The listing builds one solid part. Answer for the finished solid, in the listing's coordinates (mm). A direction names the side the tool comes from. Coordinates: 2 decimals unless noted, no trailing zeros. Order: outer loops, then holes, each group sorted by start corner. A loop starts at its lowest first (then second) coordinate and runs counter-clockwise, first axis right, second up. Notation, with made-up numbers: (-23.5, -27) -> (35.5, -27) arc R21 cw to (35.5, -22) -> close; hole circle Ø9 at (62, -14). An arc over 180 degrees is marked (long way). Return JSON: item names as keys, results as strings.
from build123d import *

# Parameters (mm, degrees)
F0_R     = 24.765
F0_R_2   = 21.082
F1_DEPTH = 30.48
F0_R_3   = 17.272
F0_R_4   = 5.55625
F2_DEPTH = 5.08
F3_SIZE2 = 4.7397045256
F3_SIZE  = 1.27
F4_SIZE  = 1.27


with BuildPart() as f1:
    # F0 (on Top) → F1 (new body)
    with BuildSketch(Plane.XY):
        Circle(F0_R)
        Circle(F0_R_2, mode=Mode.SUBTRACT)
    extrude(amount=F1_DEPTH)



with BuildPart() as f1b:
    # F0 (on Top) → F1, piece 2 (new body)
    with BuildSketch(Plane.XY):
        Circle(F0_R_3)
        Circle(F0_R_4, mode=Mode.SUBTRACT)
    extrude(amount=F1_DEPTH)


with BuildPart() as f1_1:
    add(f1.part)

    add(f1b.part)  # F2 merges F1b
    # F0 (on Top) → F2 (join)
    with BuildSketch(Plane.XY):
        Circle(F0_R_2)
        Circle(F0_R_3, mode=Mode.SUBTRACT)
    extrude(amount=F2_DEPTH)

    # F3
    f3_edges = [f1_1.edges().sort_by_distance(p)[0] for p in [
        (-24.765, 0, 30.48),
    ]]
    f3_side = f1_1.faces().sort_by_distance((-24.06454, 0, 30.48))[0]
    chamfer(f3_edges, length=F3_SIZE, length2=F3_SIZE2, reference=f3_side)

    # F4
    f4_edges = [f1_1.edges().sort_by_distance(p)[0] for p in [
        (-24.765, 0, 0),
    ]]
    chamfer(f4_edges, length=F4_SIZE)


solid = f1_1.part
1. Each of these flat-tipped pins is pushed along its axis until it touches: pin 1 Ø14.5 at (x, y) = (0, 0) entering from +Z; pin 2 Ø1.5 at (y, z) = (-15, 24.5) entering from -X; pin 3 Ø2 at (x, z) = (-17.5, 26) entering from +Y; pin 4 Ø6 at (x, z) = (-14, 5) entering from -Y. Where does it stop, or does it pass through?
Answer block:
{"pin 1": "stops at z = 30.48", "pin 2": "stops at x = -20.25", "pin 3": "stops at y = 18.44", "pin 4": "stops at y = -22.19"}
2. Determine the mould class of faces 3 (the face through (-6, 0, 0)), 4 (the face through (20.11, 6.33, 17.6)), 5 (the face through (-5.11, -23.014, 30.184)) for opening direction X: pulls with the +X half, pulls with the -X half, needs draft (parallel to the pull), parting line crosses it, or undercut.
Answer block:
{"face 3": "needs draft", "face 4": "undercut", "face 5": "parting line crosses it"}
3. The part is cut by section A-A on x = 0. Give the vertices of the cut face in (y, z) (3 decimals).
Answer block:
{"outline": "(-24.765, 1.27) -> (-23.495, 0) -> (-5.556, 0) -> (-5.556, 30.48) -> (-17.272, 30.48) -> (-17.272, 5.08) -> (-21.082, 5.08) -> (-21.082, 30.48) -> (-23.495, 30.48) -> (-24.765, 25.74) -> close; (5.556, 0) -> (23.495, 0) -> (24.765, 1.27) -> (24.765, 25.74) -> (23.495, 30.48) -> (21.082, 30.48) -> (21.082, 5.08) -> (17.272, 5.08) -> (17.272, 30.48) -> (5.556, 30.48) -> close"}
4. Consider line 1 (Y direction, x = 0, z = 17.5) (3 decimals); line 2 (X direction, y = 10.5, z = 28); line 3 (X direction, y = 10, z = 25.5). Determine where each line is inside the solid, lowest interval first. Write a range as from..to.
Answer block:
{"line 1": "y = -24.765..-21.082, -17.272..-5.556, 5.556..17.272, 21.082..24.765", "line 2": "x = -21.76..-18.28, -13.71..13.71, 18.28..21.76", "line 3": "x = -22.66..-18.56, -14.08..14.08, 18.56..22.66"}
5. The part is cut by section C-C on z = 7.5. Give the vertices of the cut face in (x, y) (1 decimal).
Answer block:
{"outline": "circle Ø49.5 at (0, 0); circle Ø34.5 at (0, 0); hole circle Ø42.2 at (0, 0); hole circle Ø11.1 at (0, 0)"}
6. For faces 1 (the face through (-8, -16, 5.08)), 2 (the face through (5.3, 1.67, 15.03)), determine the directions among +Z, -Z, +X, -X, +Y, -Y from which every point of the face is accessible in a straight line to the end or side of a thin tool.
Answer block:
{"face 1": "+Z", "face 2": "+Z, -Z"}
7. The part is cut by section D-D on z = 2.5. Give the vertices of the cut face in (x, y) (1 decimal).
Answer block:
{"outline": "circle Ø49.5 at (0, 0); hole circle Ø11.1 at (0, 0)"}
